from build123d import *

# Parameters (mm, degrees)
F0_W      = 300
F0_H      = 200
F1_DEPTH  = 300
F2_W      = 260
F2_H      = 200
F3_DEPTH  = 260
F4_R      = 10
F5_W      = 60
F5_H      = 50
F6_DEPTH  = 260
F7_SIZE   = 10
F8_W      = 60
F8_H      = 50
F9_DEPTH  = 200
F11_DEPTH = 50


# Not quite as in the source:
# - a feature names something its author has since deleted; it is built from what else it names


with BuildPart() as f1:
    # F0 (on Top) → F1 (new body)
    with BuildSketch(Plane.XY):
        with Locations((-1.4433003962, 18.309512734)):
            Rectangle(F0_W, F0_H)
    extrude(amount=F1_DEPTH)

    # F2 (on face) → F3 (cut)
    with BuildSketch(Plane.XY.offset(300)):
        with Locations((18.5566996038, 18.309512734)):
            Rectangle(F2_W, F2_H)
    extrude(amount=-F3_DEPTH, mode=Mode.SUBTRACT)

    # F4
    f4_edges = [f1.edges().sort_by_distance(p)[0] for p in [
        (-111.4433, 18.309513, 40),
    ]]
    fillet(f4_edges, radius=F4_R)

    # F5 (on face) → F6 (join)
    with BuildSketch(Plane.XY.offset(300)):
        with Locations((-81.4433003962, 15.5513301492)):
            Rectangle(F5_W, F5_H)
    extrude(amount=-F6_DEPTH)

    # F7
    f7_edges = [f1.edges().sort_by_distance(p)[0] for p in [
        (-151.4433, 18.309513, 0),
        (148.5567, -81.690487, 20),
        (148.5567, 118.309513, 20),
    ]]
    chamfer(f7_edges, length=F7_SIZE)

    # F8 (on face) → F9 (cut)
    with BuildSketch(Plane.XY.offset(300)):
        with Locations((-81.4433003962, 15.5513301492)):
            Rectangle(F8_W, F8_H)
    extrude(amount=-F9_DEPTH, mode=Mode.SUBTRACT)

    # F10 (on face) → F11 (cut)
    with BuildSketch(Plane.XZ.offset(9.4486698508)):
        Polygon((-51.4433003962, 100), (-111.4433003962, 100), (-51.4433003962, 40), align=None)
    extrude(amount=-F11_DEPTH, mode=Mode.SUBTRACT)


solid = f1.part
Source: CAD feature listing. Evaluate the final solid. Frame: model axes, mm. A direction names the side the tool comes from. Round coordinates to 2 decimals unless told otherwise and drop trailing zeros. Write each loop counter-clockwise with the first axis right and the second up, starting at its lowest first coordinate (ties: lowest second). Pieces come first, ordered by that corner, then holes. Notation, with made-up numbers: M 47,14.5 L 66,14.5 A22 cw 66,46.5 Z; hole C -30.75,56.5 d2. An arc over 180 degrees is marked long. One line per item, written item: value. Start each with the question number.
Item 1: Section query B-B (z = 66). Return the cut outline in (x, y), plus the area to 3 significant figures.
Item 2: Set-up query: faces 1 (the flat face through (-95, -9.449, 57)), 2 (the flat face through (-132, 20, 300)), 3 (the cylindrical face through (-108.436, 79.975, 42.852)). Return all of +Z, -Z, +X, -X, +Y, -Y with unobstructed straight access to the full face (end or side cutting, diameter ignored); none if empty.
Item 3: Pin query (flat end, axial travel): pin 1 (5 mm diameter, centred on y = 49.5, z = 245.5, fed in from +X); pin 2 (3 mm diameter, centred on x = 36.5, y = 90.5, fed in from +Z). Return the tip coordinate at first contact, or that it passes through.
Item 4: Section query D-D (z = 186). Return the cut outline in (x, y).
Item 5: Ray query, L1, parallel to Z at x = -84.5, y = -55.5; L2, parallel to X at y = 105, z = 170; L3, parallel to X at y = 78, z = 41. Return the intervals inside material, ascending. Write a range as from..to.
Item 6: Section query A-A (y = -1.5). Return the cut outline in (x, z), plus the area to 4 significant figures.
Item 7: Section query C-C (x = -37.5). Return the cut outline in (y, z).
Result set:
1. outline: M -151.44,-81.69 L -111.44,-81.69 L -111.44,-9.45 L -77.44,-9.45 L -77.44,40.55 L -111.44,40.55 L -111.44,118.31 L -151.44,118.31 Z
1. area: 9,700 mm²
2. face 1: +Z, +X, -Y
2. face 2: +Z, +X, -X, +Y, -Y
2. face 3: +Z, +X, +Y
3. pin 1: stops at x = -111.44
3. pin 2: stops at z = 40
4. outline: M -151.44,-81.69 L -111.44,-81.69 L -111.44,118.31 L -151.44,118.31 Z
5. L1: z = 0..40
5. L2: x = -151.44..-111.44
5. L3: x = -151.44..-105.8
6. outline: M -151.44,10 L -141.44,0 L 148.56,0 L 148.56,40 L -51.44,40 L -111.44,100 L -111.44,300 L -151.44,300 Z
6. area: 24,150 mm²
7. outline: M -81.69,0 L 118.31,0 L 118.31,40 L -81.69,40 Z
